from build123d import *

# Parameters (mm, degrees)
SKETCH1_R           = 1.65
BOSS_EXTRUDE1_DEPTH = 5
FILLET1_R           = 2.5
SKETCH2_W           = 2.5
SKETCH2_H           = 6
SKETCH2_W_2         = 30
BOSS_EXTRUDE2_DEPTH = 10
SKETCH3_R           = 2.5
CUT_EXTRUDE1_DEPTH  = 70.485517916


with BuildPart() as part:
    # Sketch1 → Boss-Extrude1 (new body)
    with BuildSketch(Plane(origin=(0, 0, 0), x_dir=(1, 0, 0), z_dir=(0, 1, 0))):
        with BuildLine():
            Line((0, -5), (-31.161412035, -5))
            ThreePointArc((-31.161412035, -5), (0, 31.56), (31.161412035, -5))
            Line((31.161412035, -5), (0, -5))
        make_face()
        with Locations(Location((0, 0, 0), (0, 0, 270))):
            Circle(SKETCH1_R, mode=Mode.SUBTRACT)
        with Locations(Location((0, 26.56, 0), (0, 0, 270))):
            Circle(SKETCH1_R, mode=Mode.SUBTRACT)
    extrude(amount=BOSS_EXTRUDE1_DEPTH)

    # Fillet1
    fillet1_edges = [part.edges().sort_by_distance(p)[0] for p in [
        (31.161412035, 2.5, 5),
        (-31.161412035, 2.5, 5),
    ]]
    fillet(fillet1_edges, radius=FILLET1_R)

    # Sketch2 → Boss-Extrude2 (add)
    with BuildSketch(Plane(origin=(0, 5, 0), x_dir=(1, 0, 0), z_dir=(0, 1, 0))):
        with Locations((-27.25, 6)):
            Rectangle(SKETCH2_W, SKETCH2_H)
        with Locations((27.25, 6)):
            Rectangle(SKETCH2_W, SKETCH2_H)
        with Locations((0, 6)):
            Rectangle(SKETCH2_W_2, SKETCH2_H)
    extrude(amount=BOSS_EXTRUDE2_DEPTH)

    # Sketch3 → Cut-Extrude1 (cut, through all)
    with BuildSketch(Plane.ZY.offset(28.5)):
        with Locations((-6, 12)):
            Circle(SKETCH3_R)
    extrude(amount=-CUT_EXTRUDE1_DEPTH, mode=Mode.SUBTRACT)


solid = part.part
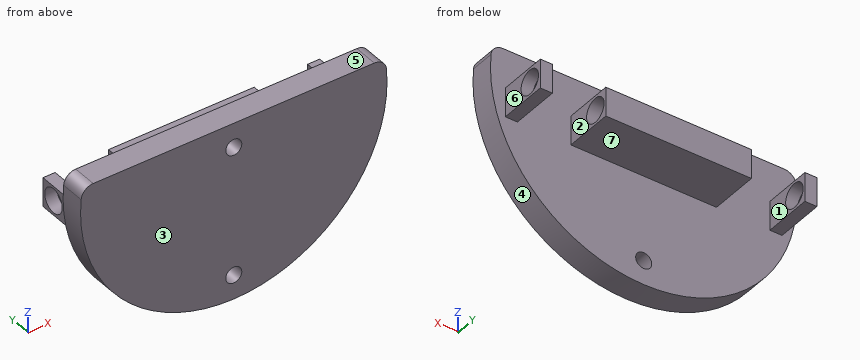
Build history of the part. All positions in model axes, mm. Face numbers are marked on the shaded views. A direction names the side the tool comes from. Round coordinates to 2 decimals unless told otherwise and drop trailing zeros. Write each loop counter-clockwise with the first axis right and the second up, starting at its lowest first coordinate (ties: lowest second). Pieces come first, ordered by that corner, then holes. Notation, with made-up numbers: M 22.5,45 L 66.5,45 A28 ccw 66.5,67 Z; hole C 3.25,19 d1. An arc over 180 degrees is marked long. Answer in a Markdown table with one row per item.
1. Which spindle directions (+Z, -Z, +X, -X, +Y, -Y) get a long thin tool onto all of the face, cutting with end or side? Do the marked faces 5, 6 and 7. Say none if no direction does.
Geometry check:
| item | result |
|---|---|
| face 5 | +Z, +X, -X, +Y, -Y |
| face 6 | +Z, -Z, +X, +Y |
| face 7 | -Z, +X, -X, +Y |
2. Flat gauge pins, fed straight in: P1, Ø2, axis at x = 27, y = 8, coming from the -Z side; P2, Ø5, axis at y = 9, z = -4.5, coming from the +X side; P3, Ø5, axis at y = 12.5, z = -6.5, coming from the -X side; P4, Ø2, axis at x = 0, z = -26.56, coming from the +Y side. Where does each tip first touch, or does it go through?
Geometry check:
| item | result |
|---|---|
| P1 | z = -9 |
| P2 | x = 28.5 |
| P3 | x = -28.5 |
| P4 | through |
3. Probe L1, parallel to Z at x = -12, y = 11.75; L2, parallel to Y at x = 4, z = -6; L3, parallel to Y at x = -8, z = -27.5. List the from-to ranges inside material, lowest first. Write a range as [from, to].
Geometry check:
| item | result |
|---|---|
| L1 | [-9, -8.49], [-3.51, -3] |
| L2 | [0, 9.5], [14.5, 15] |
| L3 | [0, 5] |
4. Saw through at D-D (z = -6). List the corners of the cut face in (x, y).
Geometry check:
| item | result |
|---|---|
| outline | M -30.98,0 L 30.98,0 L 30.98,5 L 28.5,5 L 28.5,9.5 L 26,9.5 L 26,5 L 15,5 L 15,9.5 L -15,9.5 L -15,5 L -26,5 L -26,9.5 L -28.5,9.5 L -28.5,5 L -30.98,5 Z; M -28.5,14.5 L -26,14.5 L -26,15 L -28.5,15 Z; M -15,14.5 L 15,14.5 L 15,15 L -15,15 Z; M 26,14.5 L 28.5,14.5 L 28.5,15 L 26,15 Z |
5. Mould opens along X. For the marked faces 1, 2, 3 and 4 say: +X half, -X half, draft (parallel to the pull), parting line (faces both ways), or undercut.
Geometry check:
| item | result |
|---|---|
| face 1 | undercut |
| face 2 | undercut |
| face 3 | draft |
| face 4 | parting line |
6. Saw through at B-B (y = 12). List the corners of the cut face in (x, z).
Geometry check:
| item | result |
|---|---|
| outline | M -28.5,-9 L -26,-9 L -26,-8.5 L -28.5,-8.5 Z; M -28.5,-3.5 L -26,-3.5 L -26,-3 L -28.5,-3 Z; M -15,-9 L 15,-9 L 15,-8.5 L -15,-8.5 Z; M -15,-3.5 L 15,-3.5 L 15,-3 L -15,-3 Z; M 26,-9 L 28.5,-9 L 28.5,-8.5 L 26,-8.5 Z; M 26,-3.5 L 28.5,-3.5 L 28.5,-3 L 26,-3 Z |
7. Saw through at C-C (z = 0). List the corners of the cut face in (x, y), and give its area (3 significant figures).
Geometry check:
| item | result |
|---|---|
| outline | M -31.56,0 L -1.65,0 L -1.65,5 L -31.56,5 Z; M 1.65,0 L 31.56,0 L 31.56,5 L 1.65,5 Z |
| area | 299 mm2 |
8. Saw through at A-A (x = 0). List the corners of the cut face in (y, z), and give its area (3 significant figures).
Geometry check:
| item | result |
|---|---|
| outline | M 0,-31.56 L 5,-31.56 L 5,-28.21 L 0,-28.21 Z; M 0,-24.91 L 5,-24.91 L 5,-9 L 15,-9 L 15,-3 L 5,-3 L 5,-1.65 L 0,-1.65 Z; M 0,1.65 L 5,1.65 L 5,5 L 0,5 Z; hole C 12,-6 d5 |
| area | 190 mm2 |
